from build123d import *

# Parameters (mm, degrees)
F1_DEPTH = 25.4
F2_DEPTH = 12.7
F3_R     = 6.999522
F4_DEPTH = 76.2


with BuildPart() as f1:
    # F0 (on Front) → F1 (new body, symmetric)
    with BuildSketch(Plane.XZ):
        Polygon((0, 38.1), (0, 0), (76.2, 0), (76.2, 12.7), (50.8, 12.7), (50.8, 25.969388), (25.4, 25.969388), (25.4, 51.369388), (12.7, 51.369388), align=None)
    extrude(amount=F1_DEPTH, both=True)

    # F0 (on Front) → F2 (join, symmetric)
    with BuildSketch(Plane.XZ):
        Polygon((38.1, 51.369388), (25.4, 51.369388), (25.4, 25.969388), (50.8, 25.969388), (50.8, 38.669388), (38.1, 38.669388), align=None)
    extrude(amount=F2_DEPTH, both=True)

    # F3 (on Right) → F4 (cut)
    with BuildSketch(Plane.YZ):
        with Locations((0, 12.7047)):
            Circle(F3_R)
    extrude(amount=F4_DEPTH, mode=Mode.SUBTRACT)


solid = f1.part
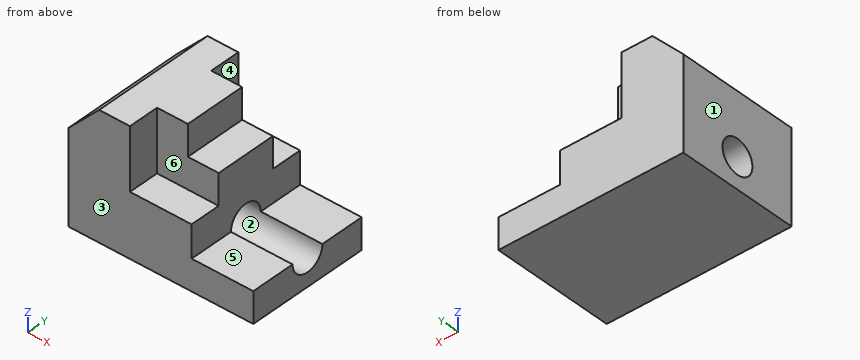
CAD build for the part. Positions are in the model's coordinates, mm. Face numbers are marked on the shaded views. A direction names the side the tool comes from. Round coordinates to 2 decimals unless told otherwise and drop trailing zeros. Write each loop counter-clockwise with the first axis right and the second up, starting at its lowest first coordinate (ties: lowest second). Pieces come first, ordered by that corner, then holes. Notation, with made-up numbers: (-6, 47.5) -> (9, 47.5) arc R19 ccw to (9, 71.5) -> close; hole circle Ø4 at (32.25, -3). An arc over 180 degrees is marked (long way). Answer as a JSON object with one key per item and string values.
(1) Pin check, flat tips, straight feed: P1, Ø20, axis at x = 59.5, y = 17.5, coming from the +Z side; P2, Ø4, axis at x = 58.5, y = 8, coming from the +Z side; P3, Ø14, axis at y = 21.5, z = 37.5, coming from the +X side. Stop position of each tip, or through.
Reported:
{"P1": "stops at z = 38.67", "P2": "stops at z = 12.7", "P3": "stops at x = 25.4"}
(2) Which spindle directions (+Z, -Z, +X, -X, +Y, -Y) get a long thin tool onto all of the face, cutting with end or side? Do the marked faces 4, 5 and 6. Say none if no direction does.
Reported:
{"face 4": "+Z, +X, +Y", "face 5": "+Z, +X, +Y, -Y", "face 6": "+Z, +X, -Y"}
(3) Probe probe 1 along Z at (x, y) = (44, 0); probe 2 along Z at (x, y) = (36, 0); probe 3 along Z at (x, y) = (64, 20.5). List the from-to ranges inside material, lowest first. Write a range as [from, to].
Reported:
{"probe 1": "z = [0, 5.71], [19.7, 38.67]", "probe 2": "z = [0, 5.71], [19.7, 51.37]", "probe 3": "z = [0, 12.7]"}
(4) Band-saw the part on D-D, the plane x = 16. List the corners of the cut face in (y, z).
Reported:
{"outline": "(-25.4, 0) -> (25.4, 0) -> (25.4, 51.37) -> (-25.4, 51.37) -> close; hole circle Ø14 at (0, 12.7)"}
(5) Band-saw the part on A-A, the plane y = 0. List the corners of the cut face in (x, z).
Reported:
{"outline": "(0, 0) -> (76.2, 0) -> (76.2, 5.71) -> (0, 5.71) -> close; (0, 19.7) -> (50.8, 19.7) -> (50.8, 38.67) -> (38.1, 38.67) -> (38.1, 51.37) -> (12.7, 51.37) -> (0, 38.1) -> close"}
(6) Band-saw the part on B-B, the plane z = 34. List the corners of the cut face in (x, y), then the cut area to 3 significant figures.
Reported:
{"outline": "(0, -25.4) -> (25.4, -25.4) -> (25.4, -12.7) -> (50.8, -12.7) -> (50.8, 12.7) -> (25.4, 12.7) -> (25.4, 25.4) -> (0, 25.4) -> close", "area": "1,940 mm^2"}
(7) Two-plate mould, pull along Y, no slides. Class the marked faces 1, 2 and 3: +Y half, -Y half, draft (parallel to the pull), parting line (faces both ways), or undercut.
Reported:
{"face 1": "draft", "face 2": "undercut", "face 3": "-Y half"}
(8) Band-saw the part on C-C, the plane y = 14.5. List the corners of the cut face in (x, z), then the cut area to 3 significant figures.
Reported:
{"outline": "(0, 0) -> (76.2, 0) -> (76.2, 12.7) -> (50.8, 12.7) -> (50.8, 25.97) -> (25.4, 25.97) -> (25.4, 51.37) -> (12.7, 51.37) -> (0, 38.1) -> close", "area": "2,200 mm^2"}
